Geometry check sheet. Reference: the model listing, model coordinates, mm. A direction names the side the tool comes from. Coordinates: 2 decimals unless noted, no trailing zeros. Write each loop counter-clockwise with the first axis right and the second up, starting at its lowest first coordinate (ties: lowest second). Pieces come first, ordered by that corner, then holes. Notation, with made-up numbers: (23, 23) -> (48, 23) arc R17 cw to (48, 54) -> close; hole circle Ø6 at (35.25, -19.75). An arc over 180 degrees is marked (long way). Answer in a Markdown table with one row per item. Add a question column.
1. Depth check by flat-ended pin: P1, Ø1, axis at x = 29, z = 6.5, coming from the +Y side (3 decimals); P2, Ø1, axis at x = 27, y = 27.5, coming from the +Z side; P3, Ø1.7, axis at x = 29, z = 115, coming from the +Y side. Enter the tip coordinate at first touch or a pass-through.
2. Mould release check, pull along Y, two halves, no side actions. Record for faces 6 (the flat face through (27.6, 20.5, 116.2)), 7 (the flat face through (27.6, 10.5, 116.2)), 8 (the flat face through (29, 10.5, 6)): pulls with the +Y half, pulls with the -Y half, needs draft (parallel to the pull), parting line crosses it, or undercut.
3. Cross-section at A-A on x = 27.2. Record the cut outline in (y, z).
4. Set-up check for faces 1 (the flat face through (29.221, 15.704, 113.672)), 2 (the flat face through (28.127, -0.205, 54.596)), 3 (the flat face through (28, 4, 112.8)), 4 (the flat face through (29, 20.5, 7)), 5 (the flat face through (28, 27, 112.8)): record each of +Z, -Z, +X, -X, +Y, -Y from which the full face is reachable in a straight line by a thin tool's end or side.
5. Scan lines: L1, parallel to Z at x = 26.9, y = 23.5; L2, parallel to Y at x = 29.65, z = 109.5; L3, parallel to Y at x = 27.45, z = 46.5. Record each from-to range of solid material in increasing order. Write a range as from..to.
6. Cross-section at C-C on z = 62.5. Record the cut outline in (x, y).
7. Cross-section at D-D on y = 6.5. Record the cut outline in (x, z).
Autodesk Inventor part; units mm, degrees
ref_plane "Work Plane3" through (0, -2, -2) normal (0, 0, -1) x (-1, 0, 0)
ref_plane "Work Plane4" through (0, 15.5, 120) normal (0, -1, 0) x (0, 0, -1)
ref_plane "YZ Plane" through (0, 0, 0) normal (1, 0, 0) x (0, 1, 0)
ref_plane "Work Plane3" through (0, -2, -2) normal (0, 0, -1) x (-1, 0, 0)
sketch "Sketch4" plane through (0, -2, -2) normal (0, 0, -1) x (-1, 0, 0)
  line L0 (-30, 33) -> (-30, 34)
  line L1 (3, -2) -> (-26, -2)
  line L2 (7, 2) -> (7, 34)
  line L3 (3, 38) -> (-26, 38)
  line L4 (-27, 17.5) -> (-42, 17.5)
  line L5 (-30, 3.2) -> (-26, 0.2)
  line L6 (-26.2, 0.2) -> (-26.2, 17.5)
  line L7 (-30, 3.2) -> (-30, 17.5)
  line L8 (-30, 31.8) -> (-26, 34.8)
  line L9 (-26.2, 34.8) -> (-26.2, 17.5)
  line L10 (-30, 31.8) -> (-30, 17.5)
  line L11 (-26.2, 3.2) -> (-25.2, 3.2)
  line L12 (-25.2, 3.2) -> (-25.2, 17.5)
  line L13 (-26.2, 31.8) -> (-25.2, 31.8)
  line L14 (-25.2, 31.8) -> (-25.2, 17.5)
  line L15 (-26, 0) -> (-30, 3)
  circle A0 centre (-11.5, 18) radius 8
  arc A1 (3, -2) -> (7, 2) centre (3, 2) ccw
  arc A2 (7, 34) -> (3, 38) centre (3, 34) ccw
  arc A3 (-26, 38) -> (-30, 34) centre (-26, 34) ccw
  line L16 (-30, 33) -> (-26, 36)
  line L17 (-26, 36) -> (-26, 0)
  line L18 (-30, 2) -> (-30, 3)
  arc A4 (-30, 2) -> (-26, -2) centre (-26, 2) ccw
  point P0 (0, 2)
  point P1 (-26.2, 0.35)
  point P2 (-26.2, 34.65)
  point P3 (-26.2, 31.8)
  point P4 (-26, 33)
  point P5 (-26, 2)
  dimension "d55" = 1
  dimension "d56" = 4
  dimension "d57" = 3
  dimension "d59" = 3.8
extrude "Whole Cover" add sketch "Sketch4" against normal blind 122 contours L9 L6 L5 L7 L10 L8
ref_plane "Work Plane4" through (0, 15.5, 120) normal (0, -1, 0) x (0, 0, -1)
sketch "Sketch5" plane through (0, 15.5, 120) normal (0, -1, 0) x (0, 0, -1)
  line L0 (122, 30) -> (0, 30)
  line L1 (122, 26.2) -> (0, 26.2)
  line L2 (0, 26.2) -> (0, 30)
  line L3 (7.85, 30) -> (-0.75, 30)
  line L4 (3.55, 30) -> (3.55, 27.8)
  line L5 (3.0945, 28.033) -> (-0.75, 30)
  line L6 (4.0055, 28.033) -> (7.85, 30)
  arc A0 (3.0945, 28.033) -> (4.0055, 28.033) centre (3.55, 28.9233) ccw
  point P0 (120, 0)
  point P1 (0, 29.6163)
  point P2 (0, 30)
  dimension "d45" = 8.6
  dimension "d47" = 2.2
  dimension "d48" = 1
extrude "Snap fit" cut sketch "Sketch5" along normal through all both and the other way through all
sketch "Sketch6" plane through (30, 1.2, -2) normal (1, 0, 0) x (0, 0, -1)
  line L0 (0, -2.85) -> (0, 31.45)
  line L1 (0, 14.3) -> (-7, 14.3) construction
  line L2 (-7, 9.3) -> (-10, 9.3)
  line L3 (-10, 9.3) -> (-10, 19.3)
  line L4 (-10, 19.3) -> (-7, 19.3)
  line L5 (-7, 19.3) -> (-7, 9.3)
  point P0 (-2, -1.2)
  dimension "d15" = 3
  dimension "d16" = 10
  dimension "d17" = 7
extrude "Grip" cut sketch "Sketch6" against normal blind 2
chamfer "Grip Chamfer" distance 1.5 angle 45 2 edges at (28, 15.5, 8) (28, 15.5, 5)
sketch "Sketch9" plane through (30, 1.2, -2) normal (1, 0, 0) x (0, 0, -1)
  line L0 (0, 0) -> (-122, 0)
  line L1 (-122, 31.45) -> (-122, -2.85)
  line L2 (-122, 14.3) -> (-114.6731, 14.3)
  line L3 (0, -2.85) -> (-122, -2.85)
  line L4 (-122, -2.85) -> (-114.5, -2.85)
  line L5 (-114.5, -2.85) -> (-114.5, 0.15)
  line L6 (-114.5, 0.15) -> (-122, 0.15)
  line L7 (-122, 0.15) -> (-122, -2.85)
  line L8 (-122, 31.45) -> (-114.5, 31.45)
  line L9 (-114.5, 31.45) -> (-114.5, 28.45)
  line L10 (-114.5, 28.45) -> (-122, 28.45)
  line L11 (-122, 28.45) -> (-122, 31.45)
  line L12 (-122, 28.45) -> (-121.6, 28.45)
  line L13 (-121.6, 28.45) -> (-121.6, 0.15)
  line L14 (-121.6, 0.15) -> (-122, 0.15)
  line L15 (-122, 0.15) -> (-122, 28.45)
  line L16 (-117.25, 0.15) -> (-117.25, -2.85)
  line L17 (-117.25, 28.45) -> (-117.25, 31.45)
  line L18 (-114.5, 9.3) -> (-122.5, 9.3)
  line L19 (-122.5, 9.3) -> (-122.5, 19.3)
  line L20 (-122.5, 19.3) -> (-114.5, 19.3)
  line L21 (-114.5, 19.3) -> (-114.5, 9.3)
  line L22 (-114.5, 0.15) -> (-114.5, 9.3)
  line L23 (-114.5, 19.3) -> (-114.5, 28.45)
  line L24 (-114.8, -2.85) -> (-114.8, 9.3)
  line L25 (-114.8, 31.45) -> (-114.8, 19.3)
  point P0 (-2, -1.2)
  point P1 (-117.25, 0)
  point P2 (-117.25, 28.6)
  point P3 (-122, 28.6)
  point P4 (-117.25, 0)
  point P5 (-114.5, 0)
  point P6 (-121.6, 9.3)
  point P7 (-121.6, 19.3)
  point P8 (-114.8, 19.3)
  dimension "d41" = 7.5
  dimension "d42" = 3
  dimension "d43" = 0.4
  dimension "d44" = 2.75
  dimension "d49" = 8
  dimension "d50" = 10
  dimension "d60" = 0.3
extrude "Corner Cut" cut sketch "Sketch9" against normal through all contours L24 L3 L16 L0 | L0 L16 L6 L24 | L16 L3 L1 L0 | L0 L1 L6 L16 | L6 L13 L18 L24 | L1 L18 L13 L6 | L18 L1 L2 L13 | L20 L13 L10 L25 | L2 L1 L20 L13 | L20 L1 L10 L13 | L10 L17 L8 L25 | L10 L1 L8 L17
fillet "Fillet5" radius 1 1 edges at (29.4116, 15.5, 119.6)
properties part number "enclosure cover_3DPrint"
Results found:
| question | item | result |
|---|---|---|
| 1 | P1 | stops at y = 30.925 |
| 1 | P2 | stops at z = 112.8 |
| 1 | P3 | stops at y = 20.5 |
| 2 | face 6 | pulls with the +Y half |
| 2 | face 7 | pulls with the -Y half |
| 2 | face 8 | undercut |
| 3 | outline | (-0.9, -2) -> (31.9, -2) -> (31.9, 112.8) -> (20.5, 112.8) -> (20.5, 119.6) -> (10.5, 119.6) -> (10.5, 112.8) -> (-0.9, 112.8) -> close |
| 4 | face 1 | +X, +Y, -Y |
| 4 | face 2 | +Z, -Z, +X, -Y |
| 4 | face 3 | +Z, +X, -X, -Y |
| 4 | face 4 | +X |
| 4 | face 5 | +Z, +X, -X, +Y |
| 5 | L1 | z = -2..112.8 |
| 5 | L2 | y = 0.94..30.06 |
| 5 | L3 | y = -0.71..31.71 |
| 6 | outline | (26.2, -1.65) -> (30, 1.2) -> (30, 29.8) -> (26.2, 32.65) -> close |
| 7 | outline | (26.2, -2) -> (30, -2) -> (30, 112.15) -> (29.67, 112.8) -> (26.2, 112.8) -> close |
